For this review, use the dimensioned drawing (mm, ordinates from the lowest corner) and the shaded views. A direction names the side the tool comes from. Give positions to 0.01 mm unless a question says otherwise; leave off trailing zeros. Order: outer loops, then holes, each group sorted by start corner. A loop starts at its lowest first (then second) coordinate and runs counter-clockwise, first axis right, second up. Notation, with made-up numbers: M 33.5,32.25 L 70.5,32.25 A29 ccw 70.5,60.25 Z; hole C 75,-29.5 d5. An arc over 180 degrees is marked long. Answer as CSV lines item,"result". Start each with the question number.
1. We need section B-B, the plane x = 9. Give the boundary of the cut face in (y, z).
2. Machinability: for the marked faces 1 and 2, which of the approach directions +Z, -Z, +X, -X, +Y, -Y give a long, thin tool a straight path to every point of the face, cutting with its end or side? Answer none if there is none.
3. For line 1 along X through (y, z) = (10, 21.5); line 2 along Y through (x, z) = (17, 26); line 3 along Z through (x, y) = (30, 1) (1 decimal), list the stretches that pass through material, from the lowest coordinate up.
4. We need section C-C, the plane z = 15. Give the boundary of the cut face in (x, y).
5. We need section A-A, the plane y = 1.5. Give the boundary of the cut face in (x, z).
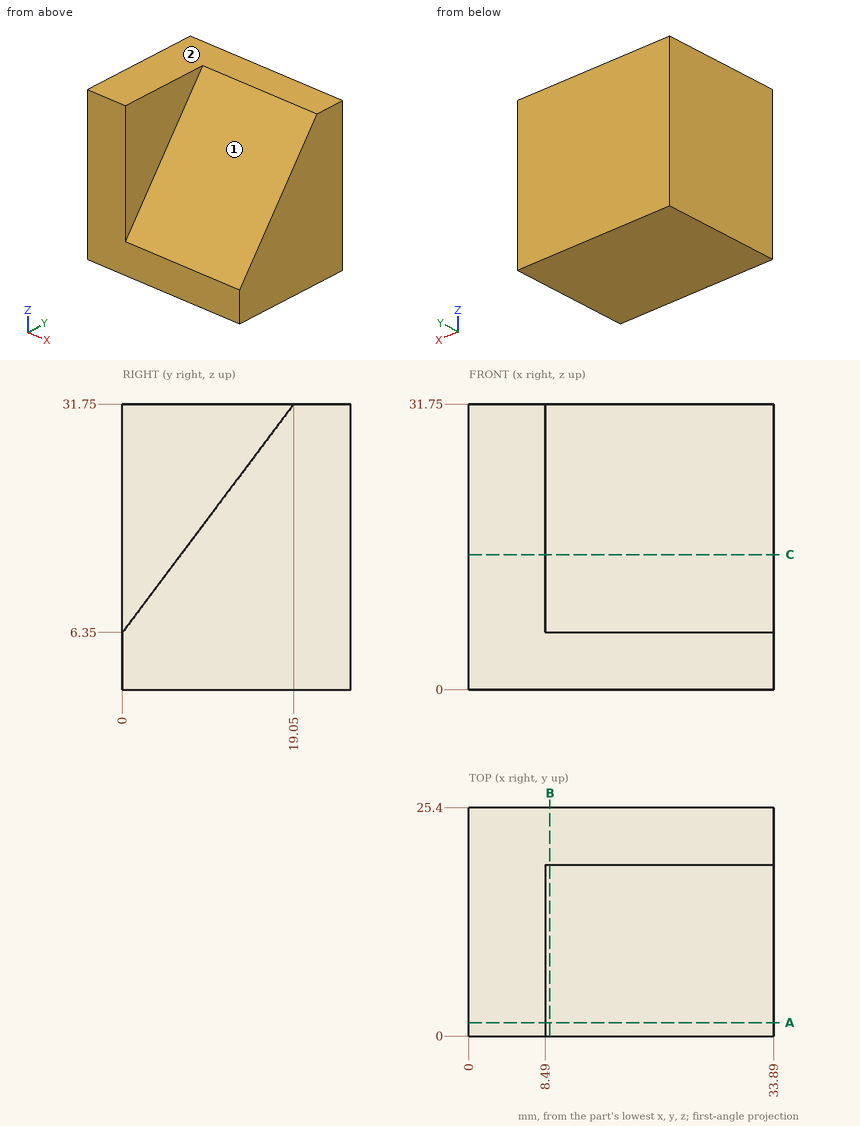
Result set:
1,outline,"M 0,0 L 25.4,0 L 25.4,31.75 L 19.05,31.75 L 0,6.35 Z"
2,face 1,"+Z, +X, -Y"
2,face 2,"+Z, +X, -X, +Y, -Y"
3,line 1,"0 to 8.49"
3,line 2,"14.74 to 25.4"
3,line 3,"0 to 7.7"
4,outline,"M 0,0 L 8.49,0 L 8.49,6.49 L 33.89,6.49 L 33.89,25.4 L 0,25.4 Z"
5,outline,"M 0,0 L 33.89,0 L 33.89,8.35 L 8.49,8.35 L 8.49,31.75 L 0,31.75 Z"
